Input: dimensioned drawing with shaded views. Units: mm. Origin: part minimum x, y, z. A direction names the side the tool comes from. Round coordinates to 2 decimals unless told otherwise and drop trailing zeros. Order: outer loops, then holes, each group sorted by start corner. A loop starts at its lowest first (then second) coordinate and runs counter-clockwise, first axis right, second up. Notation, with made-up numbers: M 6.5,-34 L 33.5,-34 A18 cw 33.5,-9 Z; hole C 37.5,83 d3. An arc over 180 degrees is marked long. Put each result on its own line as item: value. Start each with the question number.
1) Material intervals for probe 1 along X at (y, z) = (4, 5.25); probe 2 along X at (y, z) = (2.5, 18.75); probe 3 along Y at (x, z) = (13.5, 14.5) (1 decimal), sorted ascending. Write a range as [from, to].
2) Draft query along Y for the marked faces 1, 2, 3 and 4. Return one class per face: pulls with the +Y half, pulls with the -Y half, needs draft (parallel to the pull), parting line crosses it, or undercut.
3) Access query for the marked faces 5 and 6. Directions: +Z, -Z, +X, -X, +Y, -Y. A direction counts if a zero-diameter tool reaches every point of the face in a straight line with its end or side. Return the directions, or none.
4) Section D-D, the plane z = 2.5. Return loops of the section in (x, y).
5) First-contact query: P1, Ø12, axis at x = 53.5, y = 10, coming from the +Z side (1 decimal); P2, Ø0.5, axis at y = 8, z = 16.5, coming from the -X side; P3, Ø0.5, axis at x = 67.5, y = 14.5, coming from the -Z side; P4, Ø0.5, axis at x = 66, z = 20, coming from the +Y side (1 decimal). Flat tips, straight axial feed; report the tip coordinate or a pass-through.
6) Section A-A, the plane z = 15.25. Return loops of the section in (x, y) (1 decimal).
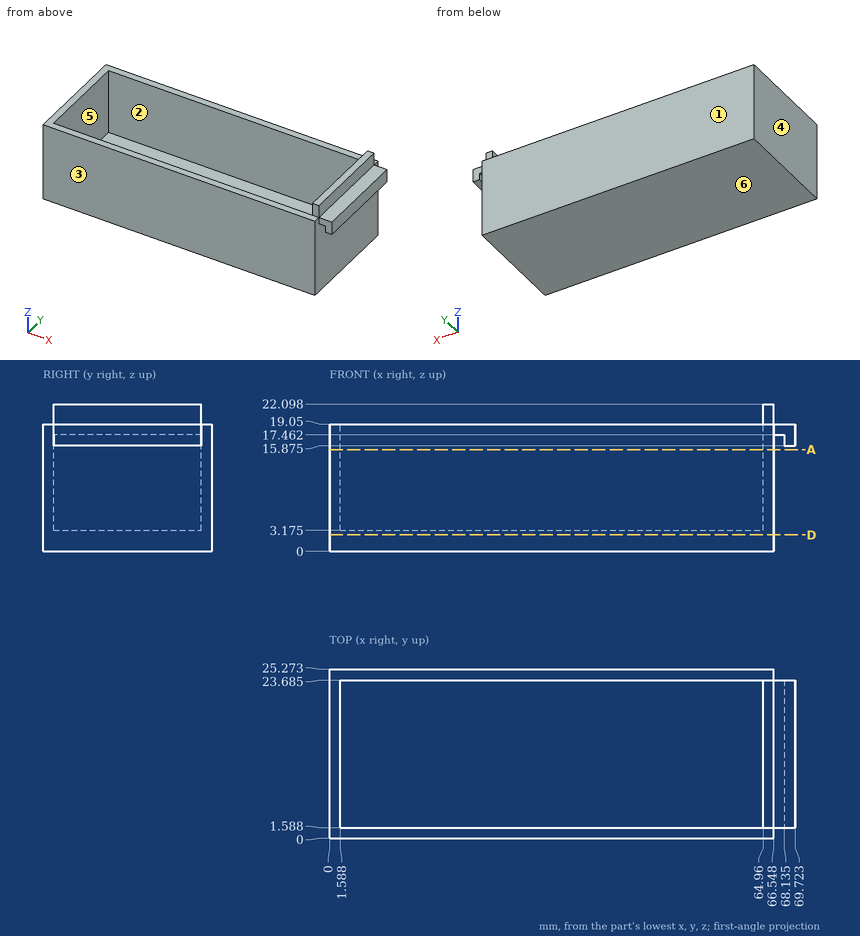
Result sheet:
1. probe 1: x = [0, 1.59], [64.96, 66.55]
1. probe 2: x = [0, 1.59], [64.96, 69.72]
1. probe 3: y = [0, 1.6], [23.7, 25.3]
2. face 1: pulls with the +Y half
2. face 2: undercut
2. face 3: pulls with the -Y half
2. face 4: needs draft
3. face 5: +Z
3. face 6: -Z, +X, -X, +Y, -Y
4. outline: M 0,0 L 66.55,0 L 66.55,25.27 L 0,25.27 Z
5. P1: stops at z = 3.2
5. P2: stops at x = 0
5. P3: stops at z = 17.46
5. P4: stops at y = 23.7
6. outline: M 0,0 L 66.5,0 L 66.5,25.3 L 0,25.3 Z; hole M 1.6,1.6 L 65,1.6 L 65,23.7 L 1.6,23.7 Z
